Source: CAD feature listing. Evaluate the final solid. Frame: model axes, mm. A direction names the side the tool comes from. Give positions to 0.01 mm unless a question says otherwise; leave off trailing zeros. Order: outer loops, then holes, each group sorted by start corner. A loop starts at its lowest first (then second) coordinate and runs counter-clockwise, first axis right, second up. Notation, with made-up numbers: (30.5, -39) - (41.5, -39) arc R7 cw to (41.5, -27) - close; hole circle Ø1 at (83.25, 80). An arc over 180 degrees is marked (long way). Write each question's results on one line, items separated by ' | '. Start each with the question number.
Item 1: Mould query, pull axis Y, two halves, no side actions, for faces 6 (the cylindrical face through (3.5, -24, -1.8)), 7 (the cylindrical face through (-0.094, -17.652, 8.758)), 8 (the flat face through (0, 0, 0)), 9 (the flat face through (0, -25.654, 0)). Classes: released by +Y, released by -Y, zero draft, split by the parting line, or undercut.
Item 2: Section D-D on x = -3.25. Output: boundary loops of the cut face in (y, z) (3 decimals), and give its area (3 significant figures).
Item 3: Section C-C on y = -5.75. Output: boundary loops of the cut face in (x, z) (3 decimals).
Item 4: Section A-A on x = 0. Output: boundary loops of the cut face in (y, z) (3 decimals).
Item 5: Line query: line 1 along Y through (x, z) = (0, -3.25); line 2 along Y through (x, z) = (4.5, 2); line 3 along X through (y, z) = (-11, 3.25). Output: solid intervals per line, ascending.
Item 6: Set-up query: faces 1 (the cylindrical face through (8.45, -12.96, -4.4)), 2 (the cylindrical face through (3.5, -1.7, -1.8)), 3 (the flat face through (-0.1, -22.352, -4.1)), 4 (the cylindrical face through (-0.17, -8.86, -0.76)), 5 (the flat face through (-2, -9, 8.255)). Return all of +Z, -Z, +X, -X, +Y, -Y with unobstructed straight access to the full face (end or side cutting, diameter ignored); none if empty.
Item 7: Section B-B on z = 0. Output: boundary loops of the cut face in (x, y) (1 decimal).
Item 8: Contact query for flat-ended pins moving along their axis: pin 1 Ø4 at (x, y) = (6, -16.5) entering from -Z; pin 2 Ø8 at (x, y) = (-6, -3) entering from +Z; pin 3 Ø2 at (x, z) = (6.5, 7) entering from +Y. Output: stop coordinate, or through.
```python
from build123d import *

# Parameters (mm, degrees)
SKETCH9_R                        = 4.826
CUT_EXTRUDE1_DEPTH               = 1.27
SKETCH10_W                       = 3.96875
SKETCH10_H                       = 17.78
F_3_8_16_TAPPED_HOLE2_AT_2_COUNT = 2
F_3_8_16_TAPPED_HOLE2_AT_2_PITCH = 29.889478418


with BuildPart() as part:
    # Sketch4 → Revolve1 (revolve)
    with BuildSketch(Plane.XY, mode=Mode.PRIVATE) as revolve1_sk:
        Polygon((0, 0), (3.937, 0), (3.937, -3.302), (9.525, -3.302), (9.525, -22.352), (3.937, -22.352), (3.937, -25.654), (0, -25.654), align=None)
    revolve(revolve1_sk.sketch.rotate(Axis((0, -25.654, 0), (0, 1, 0)), 90), axis=Axis((0, -25.654, 0), (0, 1, 0)))

    # Sketch9 → Cut-Extrude1 (cut)
    with BuildSketch(Plane.XY.offset(9.525)):
        with Locations((0, -12.827)):
            Circle(SKETCH9_R)
    extrude(amount=-CUT_EXTRUDE1_DEPTH, mode=Mode.SUBTRACT)

    # Sketch10 → 3/8-16 Tapped Hole2 (revolve, cut)
    with BuildSketch(Plane(origin=(0, -12.827, 8.255), x_dir=(0, -1, 0), z_dir=(1, 0, 0))):
        with Locations((1.984375, 8.89)):
            Rectangle(SKETCH10_W, SKETCH10_H)
    f_3_8_16_tapped_hole2 = revolve(axis=Axis((0, -12.827, 14.605), (0, 0, -1)), mode=Mode.SUBTRACT)

    # 3/8-16 Tapped Hole2 at 2: 3/8-16 Tapped Hole2 ×2
    with Locations(*[Vector(0.9929520890622513, 0.11851644960473202, 0) * (i * F_3_8_16_TAPPED_HOLE2_AT_2_PITCH) for i in range(1, F_3_8_16_TAPPED_HOLE2_AT_2_COUNT)]):
        add(f_3_8_16_tapped_hole2, mode=Mode.SUBTRACT)


solid = part.part
```
Evaluation:
1) face 6: zero draft | face 7: undercut | face 8: released by +Y | face 9: released by -Y
2) outline: (-25.654, -2.222) - (-22.352, -2.222) - (-22.352, -8.953) - (-15.105, -8.953) - (-15.105, 8.255) - (-16.395, 8.255) - (-16.395, 8.953) - (-22.352, 8.953) - (-22.352, 2.222) - (-25.654, 2.222) - close; (-10.549, -8.953) - (-3.302, -8.953) - (-3.302, -2.222) - (0, -2.222) - (0, 2.222) - (-3.302, 2.222) - (-3.302, 8.953) - (-9.259, 8.953) - (-9.259, 8.255) - (-10.549, 8.255) - close | area: 287 mm^2
3) outline: circle Ø19.05 at (0, 0)
4) outline: (-25.654, -3.937) - (-22.352, -3.937) - (-22.352, -9.525) - (-16.796, -9.525) - (-16.796, 8.255) - (-17.653, 8.255) - (-17.653, 9.525) - (-22.352, 9.525) - (-22.352, 3.937) - (-25.654, 3.937) - close; (-8.858, -9.525) - (-3.302, -9.525) - (-3.302, -3.937) - (0, -3.937) - (0, 3.937) - (-3.302, 3.937) - (-3.302, 9.525) - (-8.001, 9.525) - (-8.001, 8.255) - (-8.858, 8.255) - close
5) line 1: y = -25.65 to -16.8, -8.86 to 0 | line 2: y = -22.35 to -3.3 | line 3: x = -8.95 to -3.52, 3.52 to 8.95
6) face 1: +Y, -Y | face 2: +Y | face 3: -Y | face 4: +Z, -Z | face 5: +Z
7) outline: (-9.5, -22.4) - (-3.9, -22.4) - (-3.9, -25.7) - (3.9, -25.7) - (3.9, -22.4) - (9.5, -22.4) - (9.5, -3.3) - (3.9, -3.3) - (3.9, 0) - (-3.9, 0) - (-3.9, -3.3) - (-9.5, -3.3) - close; hole circle Ø7.9 at (0, -12.8)
8) pin 1: stops at z = -8.64 | pin 2: stops at z = 9.31 | pin 3: stops at y = -3.3
